```python
from build123d import *

# Parameters (mm, degrees)
EXTRUDE_1_DEPTH     = 0.18
CUT_EXTRUDE_1_REACH = 52.563
SKETCH_2_R          = 0.4
SKETCH_2_W          = 3
SKETCH_2_H          = 5
SKETCH_3_W          = 28
SKETCH_3_H          = 28
CUT_EXTRUDE_2_DEPTH = 0.18


with BuildPart() as part:
    # 草图1 → 凸台-拉伸1 (new body)
    with BuildSketch(Plane.XY):
        with BuildLine():
            Line((-23.82, -42.75), (23.82, -42.75))
            ThreePointArc((23.82, -42.75), (26.068599564, -41.818599564), (27, -39.57))
            Line((27, -39.57), (27, 39.57))
            ThreePointArc((27, 39.57), (26.068599564, 41.818599564), (23.82, 42.75))
            Line((23.82, 42.75), (-23.82, 42.75))
            ThreePointArc((-23.82, 42.75), (-26.068599564, 41.818599564), (-27, 39.57))
            Line((-27, 39.57), (-27, -39.57))
            ThreePointArc((-27, -39.57), (-26.068599564, -41.818599564), (-23.82, -42.75))
        make_face()
    extrude(amount=EXTRUDE_1_DEPTH)

    # 草图2 → 切除-拉伸1 (cut, up to next)
    with BuildSketch(Plane.XY.offset(0.18), mode=Mode.PRIVATE) as cut_extrude_1_sk1:
        with Locations((7.6, -21.55)):
            Circle(SKETCH_2_R)
    cut_extrude_1_tool1 = extrude(cut_extrude_1_sk1.sketch, amount=-CUT_EXTRUDE_1_REACH, mode=Mode.PRIVATE) & part.part
    # 草图2 → 切除-拉伸1 (cut, up to next)
    with BuildSketch(Plane.XY.offset(0.18), mode=Mode.PRIVATE) as cut_extrude_1_sk2:
        with Locations((12, -38.75)):
            Rectangle(SKETCH_2_W, SKETCH_2_H)
    cut_extrude_1_tool2 = extrude(cut_extrude_1_sk2.sketch, amount=-CUT_EXTRUDE_1_REACH, mode=Mode.PRIVATE) & part.part
    add(cut_extrude_1_tool1.solids().sort_by_distance((7.6, -21.55, 0.18))[0], mode=Mode.SUBTRACT)
    add(cut_extrude_1_tool2.solids().sort_by_distance((12, -38.75, 0.18))[0], mode=Mode.SUBTRACT)

    # 草图3 → 切除-拉伸2 (cut)
    with BuildSketch(Plane.XY.offset(0.18)):
        with Locations((0, 18.55)):
            Rectangle(SKETCH_3_W, SKETCH_3_H)
    extrude(amount=-CUT_EXTRUDE_2_DEPTH, mode=Mode.SUBTRACT)


solid = part.part
```
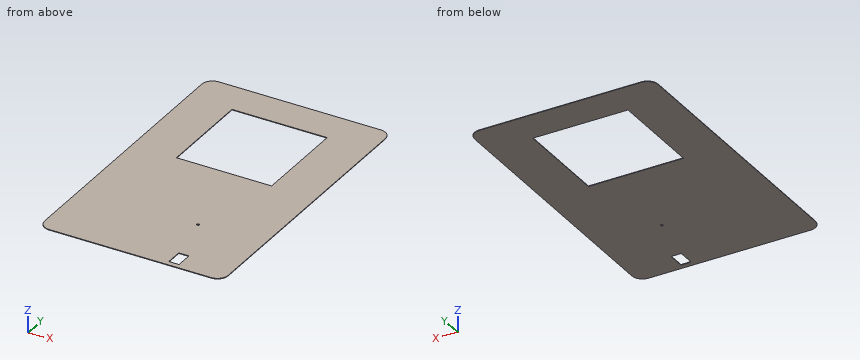
The listing builds one solid part. Answer for the finished solid, in the listing's coordinates (mm). Round coordinates to 2 decimals unless told otherwise and drop trailing zeros. Order: outer loops, then holes, each group sorted by start corner. A loop starts at its lowest first (then second) coordinate and runs counter-clockwise, first axis right, second up. Notation, with made-up numbers: (69, 41.25) -> (103, 41.25) arc R23 cw to (103, 79.25) -> close; hole circle Ø8 at (7.5, 15.25). An arc over 180 degrees is marked (long way). Answer as CSV lines item,"result".
Q1. A cutting plane is placed at B-B on x = -3.5. Determine the outline of the cut face in (y, z).
Computed values:
outline,"(-42.75, 0) -> (4.55, 0) -> (4.55, 0.18) -> (-42.75, 0.18) -> close; (32.55, 0) -> (42.75, 0) -> (42.75, 0.18) -> (32.55, 0.18) -> close"
Q2. A cutting plane is placed at A-A on y = 25. Determine the outline of the cut face in (x, z), plus the area to 3 significant figures.
Computed values:
outline,"(-27, 0) -> (-14, 0) -> (-14, 0.18) -> (-27, 0.18) -> close; (14, 0) -> (27, 0) -> (27, 0.18) -> (14, 0.18) -> close"
area,"4.68 mm^2"
Q3. Consider line 1 (Y direction, x = 7.6, z = 0.1); line 2 (X direction, y = -21.55, z = 0.1). Determine where each line is inside the solid, lowest interval first. Write a range as from..to.
Computed values:
line 1,"y = -42.75..-21.95, -21.15..4.55, 32.55..42.75"
line 2,"x = -27..7.2, 8..27"
